Could you check a few things on this model? Use its own coordinates, in mm. A direction names the side the tool comes from. Give positions to 0.01 mm unless a question says otherwise; leave off trailing zeros. Order: outer loops, then holes, each group sorted by start corner. A loop starts at its lowest first (then second) coordinate and runs counter-clockwise, first axis right, second up. Notation, with made-up numbers: M 5,29.5 L 46,29.5 A22 cw 46,66.5 Z; hole C -21.5,40 d6. An arc over 180 degrees is marked long. Use a Markdown table: item, result. Add a question column.
```python
from build123d import *

# Parameters (mm, degrees)
ESQUISSE1_R                  = 2.55
BOSS_EXTRU_1_DEPTH           = 15
ESQUISSE9_R                  = 19
BOSS_EXTRU_4_DEPTH           = 100
BOSS_EXTRU_4_DEPTH_BACK      = 23
ESQUISSE12_R                 = 9.05
ENL_V_MAT_EXTRU_2_DEPTH      = 124
ESQUISSE13_R                 = 5
ENL_V_MAT_EXTRU_3_DEPTH      = 7
ESQUISSE14_R                 = 1.5
ENL_V_MAT_EXTRU_4_DEPTH      = 32.248101798
ENL_V_MAT_EXTRU_4_DEPTH_BACK = 32.248101798
ESQUISSE15_R                 = 1.5
ENL_V_MAT_EXTRU_5_DEPTH      = 32.248101798
ENL_V_MAT_EXTRU_5_DEPTH_BACK = 32.248101798


with BuildPart() as part:
    # Esquisse1 → Boss.-Extru.1 (new body)
    with BuildSketch(Plane.XY.offset(838.2)):
        with BuildLine():
            ThreePointArc((-9.11861011, 26.177363431), (-13.892343586, 26.012514183), (-17.921893066, 28.577360682))
            ThreePointArc((-17.921893066, 28.577360682), (-29.033821851, 29.033821851), (-28.577360682, 17.921893066))
            ThreePointArc((-28.577360682, 17.921893066), (-26.012514183, 13.892343586), (-26.177363431, 9.11861011))
            ThreePointArc((-26.177363431, 9.11861011), (-19.60106383, -19.60106383), (9.11861011, -26.177363431))
            ThreePointArc((9.11861011, -26.177363431), (13.892343586, -26.012514183), (17.921893066, -28.577360682))
            ThreePointArc((17.921893066, -28.577360682), (29.033821851, -29.033821851), (28.577360682, -17.921893066))
            ThreePointArc((28.577360682, -17.921893066), (26.012514183, -13.892343586), (26.177363431, -9.11861011))
            ThreePointArc((26.177363431, -9.11861011), (19.60106383, 19.60106383), (-9.11861011, 26.177363431))
        make_face()
        with Locations((23.68807717, -23.68807717)):
            Circle(ESQUISSE1_R, mode=Mode.SUBTRACT)
        with Locations((-23.68807717, 23.68807717)):
            Circle(ESQUISSE1_R, mode=Mode.SUBTRACT)
    extrude(amount=-BOSS_EXTRU_1_DEPTH)

    # Esquisse9 → Boss.-Extru.4 (add, two sides)
    with BuildSketch(Plane.XY.offset(838.2)) as boss_extru_4_sk:
        Circle(ESQUISSE9_R)
    extrude(amount=BOSS_EXTRU_4_DEPTH)
    extrude(boss_extru_4_sk.sketch, amount=-BOSS_EXTRU_4_DEPTH_BACK)

    # Esquisse12 → Enlèv. mat.-Extru.2 (cut, through all)
    with BuildSketch(Plane.XY.offset(938.2)):
        Circle(ESQUISSE12_R)
    extrude(amount=-ENL_V_MAT_EXTRU_2_DEPTH, mode=Mode.SUBTRACT)

    # Esquisse13 → Enlèv. mat.-Extru.3 (cut)
    with BuildSketch(Plane.XY.offset(838.2)):
        with Locations((-23.68807717, 23.68807717)):
            Circle(ESQUISSE13_R)
        with Locations((23.68807717, -23.68807717)):
            Circle(ESQUISSE13_R)
    extrude(amount=-ENL_V_MAT_EXTRU_3_DEPTH, mode=Mode.SUBTRACT)

    # Esquisse14 → Enlèv. mat.-Extru.4 (cut, two sides)
    with BuildSketch(Plane(origin=(0, 0, 0), x_dir=(1, 0, 0), z_dir=(0, 1, 0))) as enl_v_mat_extru_4_sk:
        with Locations((0, -858.2)):
            Circle(ESQUISSE14_R)
        with Locations((0, -908.2)):
            Circle(ESQUISSE14_R)
    extrude(amount=ENL_V_MAT_EXTRU_4_DEPTH, mode=Mode.SUBTRACT)
    extrude(enl_v_mat_extru_4_sk.sketch, amount=-ENL_V_MAT_EXTRU_4_DEPTH_BACK, mode=Mode.SUBTRACT)

    # Esquisse15 → Enlèv. mat.-Extru.5 (cut, two sides)
    with BuildSketch(Plane(origin=(0, 0, 0), x_dir=(0, 0, -1), z_dir=(1, 0, 0))) as enl_v_mat_extru_5_sk:
        with Locations((-858.2, 0)):
            Circle(ESQUISSE15_R)
        with Locations((-908.2, 0)):
            Circle(ESQUISSE15_R)
    extrude(amount=ENL_V_MAT_EXTRU_5_DEPTH, mode=Mode.SUBTRACT)
    extrude(enl_v_mat_extru_5_sk.sketch, amount=-ENL_V_MAT_EXTRU_5_DEPTH_BACK, mode=Mode.SUBTRACT)


solid = part.part
```
1) For pin 1 (12 mm diameter, centred on y = -18.5, z = 909.5, fed in from +X); pin 2 (5 mm diameter, centred on x = 0, z = 908.2, fed in from -Y); pin 3 (3.5 mm diameter, centred on y = 0, z = 858.2, fed in from -X); pin 4 (2.5 mm diameter, centred on y = 0, z = 858.2, fed in from -X), each with a flat end and sliding along its axis, tell me the tip position at first contact or that it passes through.
2) We'd pull the mould along X, two halves only. Please class faces 1 (the face through (-14, 14, 838.2)), 2 (the face through (-0.325, -13.891, 909.664)), 3 (the face through (8.767, -16.856, 819.256)): pulls with the +X half, pulls with the -X half, needs draft (parallel to the pull), parting line crosses it, or undercut.
3) For faces 4 (the face through (-21.5, 21.5, 831.2)), 5 (the face through (-13.89, 0.07, 909.7)), which set-ups out of +Z, -Z, +X, -X, +Y, -Y let a thin tool reach every point of the face, with its end or its side?
4) Suppose I cut it at A-A on y = 0. Count the separate pieces of the cut face and the enclosed holes in it, and give its area (3 significant figures).
5) Please list where these lines run through material, in increasing order: line 1 (Z direction, x = 0, y = 14.25); line 2 (Y direction, x = 0, z = 902); line 3 (Y direction, x = -2, z = 854). Write a range as from..to.
6) Suppose I cut it at C-C on z = 908.2. Please give me the cut outline in (x, y).
7) Suppose I cut it at D-D on y = 16. Please give me the cut outline in (x, z).
Values found:
| question | item | result |
|---|---|---|
| 1 | pin 1 | stops at x = 14.31 |
| 1 | pin 2 | stops at y = -19 |
| 1 | pin 3 | stops at x = -19 |
| 1 | pin 4 | passes through |
| 2 | face 1 | needs draft |
| 2 | face 2 | undercut |
| 2 | face 3 | parting line crosses it |
| 3 | face 4 | +Z |
| 3 | face 5 | +X, -X |
| 4 | separate pieces | 6 |
| 4 | enclosed holes | 0 |
| 4 | area | 2,590 mm^2 |
| 5 | line 1 | z = 815.2..856.7, 859.7..906.7, 909.7..938.2 |
| 5 | line 2 | y = -19..-9.05, 9.05..19 |
| 5 | line 3 | y = -18.89..-8.83, 8.83..18.89 |
| 6 | outline | M -18.94,-1.5 A19 ccw -1.5,-18.94 L -1.5,-8.92 A9.05 cw -8.92,-1.5 Z; M -18.94,1.5 L -8.92,1.5 A9.05 cw -1.5,8.92 L -1.5,18.94 A19 ccw Z; M 1.5,-18.94 A19 ccw 18.94,-1.5 L 8.92,-1.5 A9.05 cw 1.5,-8.92 Z; M 1.5,8.92 A9.05 cw 8.92,1.5 L 18.94,1.5 A19 ccw 1.5,18.94 Z |
| 7 | outline | M -26.93,823.2 L -10.25,823.2 L -10.25,815.2 L 10.25,815.2 L 10.25,823.2 L 22.64,823.2 L 22.64,838.2 L 10.25,838.2 L 10.25,938.2 L -10.25,938.2 L -10.25,838.2 L -26.93,838.2 Z; hole C 0,858.2 d3; hole C 0,908.2 d3 |
